from build123d import *

# Parameters (mm, degrees)
F1_DEPTH      = 179
F2_W          = 90.0000002235
F2_H          = 169.0000002235
F3_DEPTH      = 200
F3_DEPTH_BACK = 200
F4_W          = 180.0000002235
F4_H          = 169.0000002235
F5_DEPTH      = 25


# Not quite as in the source:
# - the program builds the solid bodies; features that only make, move or delete a surface that nothing else refers to are left out


with BuildPart() as f1:
    # F0 (on Top) → F1 (new body)
    with BuildSketch(Plane.XY):
        Polygon((-74.2097248461, 100), (-74.2097248461, 0), (115.7902751539, 0), (115.7902751539, 100), (110.7902751539, 100), (110.7902751539, 5), (-69.2097248461, 5), (-69.2097248461, 100), align=None)
    extrude(amount=F1_DEPTH)

    # F2 (on face) → F3 (cut, two sides)
    with BuildSketch(Plane.YZ.offset(115.7902751539)) as f3_sk:
        with Locations((50, 89.5)):
            Rectangle(F2_W, F2_H)
    extrude(amount=F3_DEPTH, mode=Mode.SUBTRACT)
    extrude(f3_sk.sketch, amount=-F3_DEPTH_BACK, mode=Mode.SUBTRACT)

    # F4 (on face) → F5 (cut)
    with BuildSketch(Plane.XZ):
        with Locations((20.7902751539, 89.5)):
            Rectangle(F4_W, F4_H)
    extrude(amount=-F5_DEPTH, mode=Mode.SUBTRACT)


solid = f1.part
The model under review builds one solid part; all positions refer to its coordinate system, in mm. A direction names the side the tool comes from. Round coordinates to 2 decimals unless told otherwise and drop trailing zeros. Write each loop counter-clockwise with the first axis right and the second up, starting at its lowest first coordinate (ties: lowest second). Pieces come first, ordered by that corner, then holes. Notation, with made-up numbers: M 23.5,-11.5 L 75.5,-11.5 A14 cw 75.5,1.5 Z; hole C 51.5,-13 d8. An arc over 180 degrees is marked long. Answer as CSV lines item,"result". Start each with the question number.
Q1. Clearance check with flat-ended pins moving along their axes: P1, Ø1.5, axis at x = 13.5, z = 3.5, coming from the +Y side; P2, Ø10, axis at y = 89.5, z = 120, coming from the -X side. State where each tip first meets the part, or that it passes through.
Q2. The part is to be moulded in two halves that separate along Y. For faces 1 (the face through (113, 5, 88)), 2 (the face through (13, 0, 175)), 3 (the face through (-69.21, 2, 88)), say which applies: +Y half, -Y half, draft (parallel to the pull), parting line (faces both ways), or undercut.
Q3. Consider section C-C, the plane x = -47. Give the boundary of the cut face in (y, z), then the cut area to 3 significant figures.
Q4. Consider section A-A, the plane y = 84.5. Give the boundary of the cut face in (x, z).
Q5. Tool access review of faces 4 (the face through (-72, 100, 88)), 5 (the face through (20, 2, 0)), 6 (the face through (110.79, 2, 88)), 7 (the face through (-69.21, 98, 89)), 8 (the face through (-72, 49, 174)): name each direction out of +Z, -Z, +X, -X, +Y, -Y from which nothing blocks a thin tool from reaching the whole face with its end or side.
Q6. Consider section B-B, the plane z = 56. Give the boundary of the cut face in (x, y).
Result set:
1,P1,"stops at y = 5"
1,P2,"passes through"
2,face 1,"undercut"
2,face 2,"-Y half"
2,face 3,"draft"
3,outline,"M 0,0 L 5,0 L 5,5 L 0,5 Z; M 0,174 L 5,174 L 5,179 L 0,179 Z"
3,area,"50.0 mm²"
4,outline,"M -74.21,0 L -69.21,0 L -69.21,5 L -74.21,5 Z; M -74.21,174 L -69.21,174 L -69.21,179 L -74.21,179 Z; M 110.79,0 L 115.79,0 L 115.79,5 L 110.79,5 Z; M 110.79,174 L 115.79,174 L 115.79,179 L 110.79,179 Z"
5,face 4,"+Z, -Z, +X, -X, +Y"
5,face 5,"-Z, +X, -X, +Y, -Y"
5,face 6,"+Y, -Y"
5,face 7,"+Z, -Z, +Y"
5,face 8,"+X, -X"
6,outline,"M -74.21,0 L -69.21,0 L -69.21,5 L -74.21,5 Z; M -74.21,95 L -69.21,95 L -69.21,100 L -74.21,100 Z; M 110.79,0 L 115.79,0 L 115.79,5 L 110.79,5 Z; M 110.79,95 L 115.79,95 L 115.79,100 L 110.79,100 Z"
